The listing builds one solid part. Answer for the finished solid, in the listing's coordinates (mm). Round coordinates to 2 decimals unless told otherwise and drop trailing zeros. Loops run counter-clockwise (first coordinate to the right, second up) from the corner with the lowest first, then second, coordinate; pieces in that order, holes last. Notation, with made-up numbers: (24, 82.25) - (38, 82.25) arc R34 ccw to (38, 119.25) - close; hole circle Ø4 at (53, 57.25). An arc over 180 degrees is marked (long way). One line per item, written item: value.
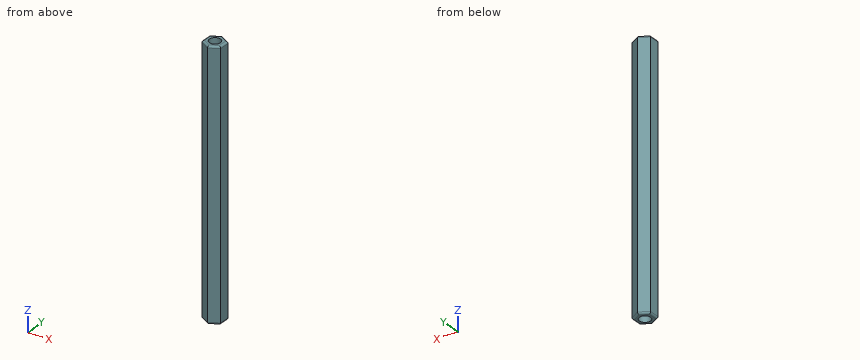
```python
from build123d import *

# Parameters (mm, degrees)
RESSALTO_EXTRUS_O1_DEPTH = 70
FILETE1_R                = 0.5
ESBO_O2_R                = 1.5
CORTE_EXTRUS_O1_DEPTH    = 71


with BuildPart() as part:
    # Esboço1 → Ressalto-extrusão1 (new body)
    with BuildSketch(Plane(origin=(0, 0, 0), x_dir=(-1, 0, 0), z_dir=(0, 0, -1))):
        Polygon((67.502122675, -1.443375673), (70.002122675, -2.886751346), (72.502122675, -1.443375673), (72.502122675, 1.443375673), (70.002122675, 2.886751346), (67.502122675, 1.443375673), align=None)
    extrude(amount=-RESSALTO_EXTRUS_O1_DEPTH)

    # Filete1
    filete1_edges = [part.edges().sort_by_distance(p)[0] for p in [
        (-71.252122675, -2.165063509, 70),
        (-72.502122675, 0, 70),
        (-71.252122675, 2.165063509, 70),
        (-68.752122675, 2.165063509, 70),
        (-67.502122675, 0, 70),
        (-68.752122675, 2.165063509, 0),
        (-71.252122675, 2.165063509, 0),
        (-72.502122675, 0, 0),
        (-71.252122675, -2.165063509, 0),
        (-68.752122675, -2.165063509, 0),
        (-67.502122675, 0, 0),
        (-68.752122675, -2.165063509, 70),
    ]]
    fillet(filete1_edges, radius=FILETE1_R)

    # Esboço2 → Corte-extrusão1 (cut, through all)
    with BuildSketch(Plane.XY.offset(70)):
        with Locations((-70.002122675, 0)):
            Circle(ESBO_O2_R)
    extrude(amount=-CORTE_EXTRUS_O1_DEPTH, mode=Mode.SUBTRACT)


solid = part.part
```
1) A cutting plane is placed at A-A on y = 0. Give the vertices of the cut face in (x, z), and give its area (3 significant figures).
Final values:
outline: (-72.5, 0.5) arc R0.5 ccw to (-72, 0) - (-71.5, 0) - (-71.5, 70) - (-72, 70) arc R0.5 ccw to (-72.5, 69.5) - close; (-68.5, 0) - (-68, 0) arc R0.5 ccw to (-67.5, 0.5) - (-67.5, 69.5) arc R0.5 ccw to (-68, 70) - (-68.5, 70) - close
area: 140 mm2
2) Consider L1, parallel to Y at x = -69.4, z = 20; L2, parallel to Y at x = -70.05, z = 8.5; L3, parallel to X at y = 0.95, z = 62. Determine where each line is inside the solid, lowest interval first.
Final values:
L1: -2.54 to -1.37, 1.37 to 2.54
L2: -2.86 to -1.5, 1.5 to 2.86
L3: -72.5 to -71.16, -68.84 to -67.5
3) This flat-tipped pin is pushed along its axis until it touches: pin 1 Ø1.5 at (x, y) = (-72, 2) entering from -Z. Where does it stop, or does it pass through?
Final values:
pin 1: z = 0
4) A cutting plane is placed at B-B on z = 34.5. Give the vertices of the cut face in (x, y).
Final values:
outline: (-72.5, -1.44) - (-70, -2.89) - (-67.5, -1.44) - (-67.5, 1.44) - (-70, 2.89) - (-72.5, 1.44) - close; hole circle Ø3 at (-70, 0)
